Autodesk Inventor part; units mm, degrees
ref_plane "YZ Plane" through (0, 0, 0) normal (1, 0, 0) x (0, 1, 0)
ref_plane "XZ Plane" through (0, 0, 0) normal (0, 1, 0) x (-1, 0, 0)
ref_plane "XY Plane" through (0, 0, 0) normal (0, 0, 1) x (1, 0, 0)
sketch "Sketch1" plane through (0, 0, 0) normal (0, 0, 1) x (1, 0, 0)
  line L0 (-72.7046, 193.4128) -> (-72.7046, 91.8128)
  line L1 (-72.7046, 193.4128) -> (130.4954, 193.4128)
  line L2 (130.4954, 193.4128) -> (130.4954, -9.7872)
  line L3 (130.4954, -9.7872) -> (28.8954, -9.7872)
  line L4 (28.8954, -9.7872) -> (-72.7046, 91.8128)
  point P0 (0, 0)
  dimension "d0" = 101.6
  dimension "d1" = 101.6
  dimension "d2" = 203.2
  dimension "d3" = 203.2
extrude "Extrusion1" add sketch "Sketch1" along normal blind 4.7625
sketch "Sketch2" plane through (0, 0, 4.7625) normal (0, 0, 1) x (1, 0, 0)
  line L0 (-72.7046, 193.4128) -> (-72.7046, 91.8128)
  line L1 (28.8954, -9.7872) -> (130.4954, -9.7872)
  line L2 (130.4954, -9.7872) -> (130.4954, 193.4128)
  line L3 (130.4954, 193.4128) -> (-72.7046, 193.4128)
  point P0 (0, 0)
  point P1 (-60.0046, 180.7128)
  point P2 (-34.6046, 180.7128)
  point P3 (-60.0046, 155.3128)
  point P4 (-34.6046, 155.3128)
  point P5 (-60.0046, 129.9128)
  point P6 (-34.6046, 129.9128)
  point P7 (-60.0046, 104.5128)
  point P8 (-34.6046, 104.5128)
  point P9 (117.7954, 79.1128)
  point P10 (117.7954, 53.7128)
  point P11 (92.3954, 79.1128)
  point P12 (92.3954, 53.7128)
  point P13 (-9.2046, 180.7128)
  point P14 (-9.2046, 155.3128)
  point P15 (-9.2046, 129.9128)
  point P16 (-9.2046, 104.5128)
  point P17 (16.1954, 180.7128)
  point P18 (16.1954, 155.3128)
  point P19 (16.1954, 129.9128)
  point P20 (16.1954, 104.5128)
  point P21 (41.5954, 180.7128)
  point P22 (41.5954, 155.3128)
  point P23 (41.5954, 129.9128)
  point P24 (41.5954, 104.5128)
  point P25 (66.9954, 180.7128)
  point P26 (66.9954, 155.3128)
  point P27 (66.9954, 129.9128)
  point P28 (66.9954, 104.5128)
  point P29 (92.3954, 180.7128)
  point P30 (92.3954, 155.3128)
  point P31 (92.3954, 129.9128)
  point P32 (92.3954, 104.5128)
  point P33 (117.7954, 180.7128)
  point P34 (117.7954, 155.3128)
  point P35 (117.7954, 129.9128)
  point P36 (117.7954, 104.5128)
  point P37 (117.7954, 28.3128)
  point P38 (92.3954, 28.3128)
  point P39 (117.7954, 2.9128)
  point P40 (92.3954, 2.9128)
  point P41 (66.9954, 79.1128)
  point P42 (66.9954, 53.7128)
  point P43 (66.9954, 28.3128)
  point P44 (66.9954, 2.9128)
  point P45 (41.5954, 79.1128)
  point P46 (41.5954, 53.7128)
  point P47 (41.5954, 28.3128)
  point P48 (41.5954, 2.9128)
  dimension "d8" = 25.4
  dimension "d11" = 25.4
  dimension "d17" = 25.4
  dimension "d20" = 25.4
  dimension "d26" = 12.7
  dimension "d27" = 12.7
  dimension "d28" = 25.4
hole "Hole1" at (-60.0046, 180.7128, 4.7625) at (-34.6046, 180.7128, 4.7625) at (-60.0046, 155.3128, 4.7625) at (-34.6046, 155.3128, 4.7625) at (-60.0046, 129.9128, 4.7625) at (-34.6046, 129.9128, 4.7625) at (-60.0046, 104.5128, 4.7625) at (-34.6046, 104.5128, 4.7625) at (117.7954, 79.1128, 4.7625) at (117.7954, 53.7128, 4.7625) at (92.3954, 79.1128, 4.7625) at (92.3954, 53.7128, 4.7625) at (-9.2046, 180.7128, 4.7625) at (-9.2046, 155.3128, 4.7625) at (-9.2046, 129.9128, 4.7625) at (-9.2046, 104.5128, 4.7625) at (16.1954, 180.7128, 4.7625) at (16.1954, 155.3128, 4.7625) at (16.1954, 129.9128, 4.7625) at (16.1954, 104.5128, 4.7625) at (41.5954, 180.7128, 4.7625) at (41.5954, 155.3128, 4.7625) at (41.5954, 129.9128, 4.7625) at (41.5954, 104.5128, 4.7625) at (66.9954, 180.7128, 4.7625) at (66.9954, 155.3128, 4.7625) at (66.9954, 129.9128, 4.7625) at (66.9954, 104.5128, 4.7625) at (92.3954, 180.7128, 4.7625) at (92.3954, 155.3128, 4.7625) at (92.3954, 129.9128, 4.7625) at (92.3954, 104.5128, 4.7625) at (117.7954, 180.7128, 4.7625) at (117.7954, 155.3128, 4.7625) at (117.7954, 129.9128, 4.7625) at (117.7954, 104.5128, 4.7625) at (117.7954, 28.3128, 4.7625) at (92.3954, 28.3128, 4.7625) at (117.7954, 2.9128, 4.7625) at (92.3954, 2.9128, 4.7625) at (66.9954, 79.1128, 4.7625) at (66.9954, 53.7128, 4.7625) at (66.9954, 28.3128, 4.7625) at (66.9954, 2.9128, 4.7625) at (41.5954, 79.1128, 4.7625) at (41.5954, 53.7128, 4.7625) at (41.5954, 28.3128, 4.7625) at (41.5954, 2.9128, 4.7625) direction (0, 0, -1) diameter 6.35 end through all
equation "\"d1\" = d0"
equation "\"d3\" = d2"
properties part number "2040-2040_mounting_plate"
The listing builds one solid part. Answer for the finished solid, in the listing's coordinates (mm). Give positions to 0.01 mm unless a question says otherwise; leave off trailing zeros. Loops run counter-clockwise (first coordinate to the right, second up) from the corner with the lowest first, then second, coordinate; pieces in that order, holes last. Notation, with made-up numbers: (73, 9.25) - (103, 9.25) arc R16 cw to (103, 31.25) - close; hole circle Ø11 at (72.25, 11). An arc over 180 degrees is marked (long way). Return JSON: item names as keys, results as strings. Group by question number.
1. Find section C-C (y = 39). Write down the section's boundary in (x, z).
2. Find section A-A (x = -1). Write down the section's boundary in (y, z).
3. Find section B-B (z = 3.25). State how many separate pieces and enclosed holes the cut face has, then the cut area to 3 significant figures.
4. Straight lines are drawn through the part: line 1 (X direction, y = 78.5, z = 2.5); line 2 (Y direction, x = 14, z = 1.6); line 3 (X direction, y = 80, z = 2.95). For each, find the intervals that lie inside material, in ascending order. Write a range as [from, to].
5. Given pin 1 Ø2 at (y, z) = (65, 1.5) entering from -X; pin 2 Ø10 at (x, y) = (41.6, 104.51) entering from +Z; pin 3 Ø2 at (x, z) = (-14, 3) entering from -Y, each flat-ended and moving along its own axis, determine where each tip first touches the part or whether it passes through.
Verdict:
{
 "1": {"outline": "(-19.89, 0) - (130.5, 0) - (130.5, 4.76) - (-19.89, 4.76) - close"},
 "2": {"outline": "(20.11, 0) - (193.41, 0) - (193.41, 4.76) - (20.11, 4.76) - close"},
 "3": {"separate pieces": "1", "enclosed holes": "48", "area": "34,600 mm^2"},
 "4": {"line 1": "x = [-59.39, 38.48], [44.71, 63.88], [70.11, 89.28], [95.51, 114.68], [120.91, 130.5]", "line 2": "y = [5.11, 102.22], [106.81, 127.62], [132.21, 153.02], [157.61, 178.42], [183.01, 193.41]", "line 3": "x = [-60.89, 38.55], [44.64, 63.95], [70.04, 89.35], [95.44, 114.75], [120.84, 130.5]"},
 "5": {"pin 1": "stops at x = -46.89", "pin 2": "stops at z = 4.76", "pin 3": "stops at y = 32.11"}
}
